from build123d import *

# Parameters (mm, degrees)
F0_W      = 124.1378337145
F0_H      = 39.50663656
F1_DEPTH  = 3
F2_W      = 2.5017783046
F2_H      = 39.50663656
F2_W_2    = 2.1480806172
F3_DEPTH  = 17.78
F5_DEPTH  = 17.78
F7_D      = 2.54
F8_W      = 30.6726247072
F8_H      = 35.56
F8_W_2    = 18.1720815599
F8_W_3    = 70.4594738781
F9_DEPTH  = 2
F11_DEPTH = 2
F13_DEPTH = 2
F15_DEPTH = 2
F16_W     = 2.9533728957
F16_H     = 20.0437232852
F16_W_2   = 2.1480806172
F16_H_2   = 20.0032039857
F16_W_3   = 2.0457915962
F17_DEPTH = 2


with BuildPart() as f1:
    # F0 (on Top) → F1 (new body)
    with BuildSketch(Plane.XY):
        Rectangle(F0_W, F0_H)
    extrude(amount=F1_DEPTH)

    # F2 (on face) → F3 (join)
    with BuildSketch(Plane.XY.offset(3)):
        with Locations((42.4621514976, 0)):
            Rectangle(F2_W, F2_H)
        with Locations((-30.3222518414, 0)):
            Rectangle(F2_W_2, F2_H)
    extrude(amount=F3_DEPTH)

    # F5 (add): faces of the model
    f5_faces = [f1.faces().sort_by_distance(p)[0] for p in [
        (-30.3222518414, 0, 20.78),
        (42.4621514976, 0, 20.78),
    ]]
    extrude(f5_faces, amount=F5_DEPTH)

    # F7 (through all)
    with Locations(Plane(origin=(-31.39629215, 0, 0), x_dir=(0, -1, 0), z_dir=(-1, 0, 0))):
        with Locations((-11.8883280084, 20.8021104336), (-15.7889463007, 20.7917392254), (-7.8511117026, 20.7805093378), (-3.6703720689, 20.7868441939)):
            Hole(F7_D / 2)

    # F8 (on face) → F9 (join)
    with BuildSketch(Plane.XZ.offset(19.75331828)):
        Polygon((-62.0689168572, 3), (-62.0689168572, 0), (61.8851222098, 0), (61.8851222098, 3), (43.7130406499, 3), (43.7130406499, 38.56), (41.2112623453, 38.56), (41.2112623453, 3), (-29.2482115328, 3), (-29.2482115328, 38.56), (-31.39629215, 38.56), (-31.39629215, 3), align=None)
        with Locations((-46.7326045036, 20.78)):
            Rectangle(F8_W, F8_H)
        with Locations((52.7990814298, 20.78)):
            Rectangle(F8_W_2, F8_H)
        with Locations((5.9815254062, 20.78)):
            Rectangle(F8_W_3, F8_H)
    extrude(amount=F9_DEPTH)

    # F10 (on face) → F11 (join)
    with BuildSketch(Plane(origin=(0, 19.75331828, 0), x_dir=(-1, 0, 0), z_dir=(0, 1, 0))):
        Polygon((-62.0689168572, 38.6005192995), (-62.0689168572, 3), (-43.7130406499, 3), (-43.7130406499, 38.56), (-41.2112623453, 38.56), (-41.2112623453, 3), (29.2482115328, 3), (29.2482115328, 38.56), (31.39629215, 38.56), (31.39629215, 3), (62.0689168572, 3), (62.0689168572, 38.6005192995), align=None)
        Polygon((-62.0689168572, 3), (-62.0689168572, 0), (62.0689168572, 0), (62.0689168572, 3), (31.39629215, 3), (31.39629215, 38.56), (29.2482115328, 38.56), (29.2482115328, 3), (-41.2112623453, 3), (-41.2112623453, 38.56), (-43.7130406499, 38.56), (-43.7130406499, 3), align=None)
    extrude(amount=F11_DEPTH)

    # F12 (on face) → F13 (join)
    with BuildSketch(Plane.YZ.offset(62.0689168572)):
        Polygon((19.75331828, 3), (19.75331828, 38.6005192995), (-22.0371708274, 38.6005192995), (-22.0371708274, 0), (-19.75331828, 0), (-19.75331828, 3), align=None)
        Polygon((21.75331828, 0), (21.75331828, 38.6005192995), (19.75331828, 38.6005192995), (19.75331828, 3), (-19.75331828, 3), (-19.75331828, 0), align=None)
    extrude(amount=F13_DEPTH)

    # F14 (on face) → F15 (join)
    with BuildSketch(Plane(origin=(-62.0689168572, 0, 0), x_dir=(0, -1, 0), z_dir=(-1, 0, 0))):
        Polygon((-21.75331828, 0), (21.75331828, 0), (21.75331828, 38.56), (19.75331828, 38.56), (19.75331828, 3), (-19.75331828, 3), (-19.75331828, 38.6005192995), (-21.75331828, 38.6005192995), align=None)
        Polygon((19.75331828, 38.56), (21.75331828, 38.56), (21.75331828, 38.6005192995), (-19.75331828, 38.6005192995), (-19.75331828, 3), (19.75331828, 3), align=None)
    extrude(amount=F15_DEPTH)

    # F16 (on face) → F17 (join)
    with BuildSketch(Plane.XZ.offset(-19.75331828)):
        with Locations((39.7345758975, 28.5786576569)):
            Rectangle(F16_W, F16_H)
        with Locations((-30.3222518414, 28.5583980072)):
            Rectangle(F16_W_2, F16_H_2)
        Polygon((-33.4356613457, 18.5567960143), (-31.39629215, 18.5567960143), (-31.39629215, 38.56), (-31.39629215, 38.6005192995), (-33.4356613457, 38.6005192995), align=None)
        Polygon((-29.2482115328, 38.56), (-29.2482115328, 18.5567960143), (-27.0928554237, 18.5567960143), (-27.0928554237, 38.6005192995), (-29.2482115328, 38.6005192995), align=None)
        with Locations((44.735936448, 28.5786576569)):
            Rectangle(F16_W_3, F16_H)
    extrude(amount=F17_DEPTH)


solid = f1.part
Model file for the job. Use its own axes, mm. A direction names the side the tool comes from. Coordinates: 2 decimals unless noted, no trailing zeros. Loops run counter-clockwise (first coordinate to the right, second up) from the corner with the lowest first, then second, coordinate; pieces in that order, holes last. Notation, with made-up numbers: (65, -19.5) -> (87, -19.5) arc R16 cw to (87, -15.5) -> close; hole circle Ø8 at (60.25, 34). An arc over 180 degrees is marked (long way). Use one line per item in the form item = value. Start each with the question number.
(1) Cut at B-B on y = -8. Give the cut face in (x, z), and give its area (3 significant figures).
(2) Probe probe 1 along X at (y, z) = (-12.5, 19.5); probe 2 along Y at (x, z) = (-2, 35); probe 3 along Z at (x, y) = (26, 3). List the from-to ranges inside material, lowest first. Write a range as from..to.
(3) Cut at D-D on z = 10. Give the cut face in (x, y), and give its area (3 significant figures).
(4) Tool access for faces 5 (the flat face through (0, -21.753, 19)), 6 (the cylindrical face through (-30.307, 12.474, 19.675)), 7 (the flat face through (40, 17.753, 29)): list every direction of +Z, -Z, +X, -X, +Y, -Y with a clear straight run to the whole face (end or side of a thin tool).
(5) Flat gauge pins, fed straight in: pin 1 (5 mm diameter, centred on x = 42, y = 11, fed in from +Z); pin 2 (8 mm diameter, centred on x = 43, z = 9, fed in from -Y). Where does each tip first touch, or does it go through?
(6) Cut at A-A on z = 36. Give the cut face in (x, y).
(7) Pull direction Z, two halves, no side cores. Call faces 1 (the cylindrical face through (42.48, 15.514, 19.552)), 2 (the flat face through (1, 0, 0)), 3 (the flat face through (0, 21, 38.601)), 4 (the cylindrical face through (42.48, 12.474, 19.675)): pulls with the +Z half, pulls with the -Z half, needs draft (parallel to the pull), parting line crosses it, or undercut.
(8) Cut at C-C on x = -3.5. Give the cut face in (y, z), and give its area (3 significant figures).
Values:
q1.outline = (-64.07, 0) -> (64.07, 0) -> (64.07, 38.6) -> (62.07, 38.6) -> (62.07, 3) -> (43.71, 3) -> (43.71, 38.56) -> (41.21, 38.56) -> (41.21, 3) -> (-29.25, 3) -> (-29.25, 38.56) -> (-31.4, 38.56) -> (-31.4, 3) -> (-62.07, 3) -> (-62.07, 38.6) -> (-64.07, 38.6) -> close
q1.area = 692 mm2
q2.probe_1 = -64.07..-62.07, -31.4..-29.25, 41.21..43.71, 62.07..64.07
q2.probe_2 = -21.75..-19.75, 19.75..21.75
q2.probe_3 = 0..3
q3.outline = (-64.07, -21.75) -> (61.89, -21.75) -> (61.89, -19.75) -> (43.71, -19.75) -> (43.71, 19.75) -> (62.07, 19.75) -> (62.07, -22.04) -> (64.07, -22.04) -> (64.07, 21.75) -> (-64.07, 21.75) -> close; hole (-62.07, -19.75) -> (-31.4, -19.75) -> (-31.4, 19.75) -> (-62.07, 19.75) -> close; hole (-29.25, -19.75) -> (41.21, -19.75) -> (41.21, 19.75) -> (-29.25, 19.75) -> close
q3.area = 854 mm2
q4.face_5 = +Z, -Z, -X, -Y
q4.face_6 = none
q4.face_7 = +Z
q5.pin_1 = 38.56
q5.pin_2 = -21.75
q6.outline = (-64.07, -21.75) -> (61.89, -21.75) -> (61.89, -19.75) -> (43.71, -19.75) -> (43.71, 17.75) -> (45.76, 17.75) -> (45.76, 19.75) -> (62.07, 19.75) -> (62.07, -22.04) -> (64.07, -22.04) -> (64.07, 21.75) -> (-64.07, 21.75) -> close; hole (-62.07, -19.75) -> (-31.4, -19.75) -> (-31.4, 17.75) -> (-33.44, 17.75) -> (-33.44, 19.75) -> (-62.07, 19.75) -> close; hole (-29.25, -19.75) -> (41.21, -19.75) -> (41.21, 17.75) -> (38.26, 17.75) -> (38.26, 19.75) -> (-27.09, 19.75) -> (-27.09, 17.75) -> (-29.25, 17.75) -> close
q7.face_1 = undercut
q7.face_2 = pulls with the -Z half
q7.face_3 = pulls with the +Z half
q7.face_4 = undercut
q8.outline = (-21.75, 0) -> (21.75, 0) -> (21.75, 38.6) -> (19.75, 38.6) -> (19.75, 3) -> (-19.75, 3) -> (-19.75, 38.56) -> (-21.75, 38.56) -> close
q8.area = 273 mm2
